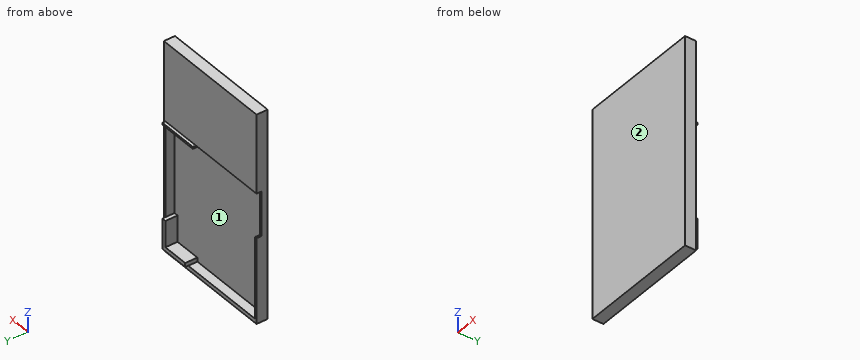
Autodesk Inventor part; units mm, degrees
ref_plane "YZ Plane" through (0, 0, 0) normal (1, 0, 0) x (0, 1, 0)
ref_plane "XZ Plane" through (0, 0, 0) normal (0, 1, 0) x (-1, 0, 0)
ref_plane "XY Plane" through (0, 0, 0) normal (0, 0, 1) x (1, 0, 0)
sketch "Sketch1" plane through (0, 0, 0) normal (0, 1, 0) x (-1, 0, 0)
  line L0 (32.9806, 40.5565) -> (-27.7594, 40.5565)
  line L1 (-27.7594, 40.5565) -> (-27.7594, -62.7415)
  line L2 (-27.7594, -62.7415) -> (32.9806, -62.7415)
  line L3 (32.9806, -62.7415) -> (32.9806, 40.5565)
  point P0 (0, 0)
  dimension "d0" = 60.74
  dimension "d1" = 103.298
extrude "Extrusion1" add sketch "Sketch1" along normal blind 1
sketch "Sketch2" plane through (0, 1, 0) normal (0, 1, 0) x (1, 0, 0)
  line L0 (-32.9806, 62.7415) -> (-32.9806, -40.5565)
  line L1 (27.7594, -40.5565) -> (27.7594, 62.7415)
  line L2 (-32.9806, -40.5565) -> (27.7594, -40.5565)
  line L3 (27.7594, -40.5565) -> (27.7594, -1.5565)
  line L4 (27.7594, -1.5565) -> (-32.9806, -1.5565)
  line L5 (-32.9806, -1.5565) -> (-32.9806, -40.5565)
  point P0 (0, 0)
  point P1 (-32.9806, -1.5565)
  dimension "d4" = 39
extrude "Extrusion2" add sketch "Sketch2" along normal blind 4.5
sketch "Sketch3" plane through (0, 1, 0) normal (0, 1, 0) x (1, 0, 0)
  line L0 (27.7594, -1.5565) -> (-32.9806, -1.5565)
  line L1 (27.7594, 62.7415) -> (-32.9806, 62.7415)
  line L2 (-32.9806, -1.5565) -> (-31.9806, -1.5565)
  line L3 (-31.9806, -1.5565) -> (-31.9806, 62.7415)
  line L4 (-31.9806, 62.7415) -> (-32.9806, 62.7415)
  line L5 (-32.9806, 62.7415) -> (-32.9806, -1.5565)
  line L6 (-31.9806, 62.7415) -> (27.7594, 62.7415)
  line L7 (27.7594, 62.7415) -> (27.7594, 60.7415)
  line L8 (27.7594, 60.7415) -> (-31.9806, 60.7415)
  line L9 (-31.9806, 60.7415) -> (-31.9806, 62.7415)
  line L10 (27.7594, -40.5565) -> (27.7594, 62.7415)
  line L11 (27.7594, -1.5565) -> (26.7594, -1.5565)
  line L12 (26.7594, -1.5565) -> (26.7594, 60.7415)
  line L13 (26.7594, 60.7415) -> (27.7594, 60.7415)
  line L14 (27.7594, 60.7415) -> (27.7594, -1.5565)
  line L15 (-32.9806, -1.5565) -> (-31.9806, -1.5565)
  line L16 (-31.9806, -1.5565) -> (-31.9806, 20.4435)
  line L17 (-31.9806, 20.4435) -> (-32.9806, 20.4435)
  line L18 (-32.9806, 20.4435) -> (-32.9806, -1.5565)
  point P0 (0, 0)
  point P1 (27.2594, -1.5565)
  point P2 (-31.9806, 60.7415)
  point P3 (-32.4806, -1.5565)
  point P4 (-32.4806, 20.4435)
  dimension "d7" = 1
  dimension "d8" = 2
  dimension "d9" = 1
  dimension "d10" = 0
  dimension "d13" = 22
extrude "Extrusion3" add sketch "Sketch3" along normal blind 4.5 contours L0 L12 L8 L10 | L8 L3 L1 L7 | L17 L5 L1 L3
sketch "Sketch4" plane through (0, 1, 0) normal (0, 1, 0) x (1, 0, 0)
  line L0 (-32.9806, 62.7415) -> (-32.9806, -40.5565)
  line L1 (-31.9806, 20.4435) -> (-32.9806, 20.4435)
  line L2 (-32.9806, 20.4435) -> (-32.9806, -2.617)
  line L3 (-32.9806, -2.617) -> (-31.9806, -2.617)
  line L4 (-31.9806, -2.617) -> (-31.9806, 20.4435)
  point P0 (0, 0)
extrude "Extrusion4" add sketch "Sketch4" along normal blind 2
sketch "Sketch5" plane through (0, 1, 0) normal (0, 1, 0) x (1, 0, 0)
  line L0 (26.7594, 60.7415) -> (26.7594, -1.5565)
  line L1 (26.7594, 60.7415) -> (11.7594, 60.7415)
  line L2 (11.7594, 60.7415) -> (11.7594, 58.7415)
  line L3 (11.7594, 58.7415) -> (26.7594, 58.7415)
  line L4 (26.7594, 58.7415) -> (26.7594, 60.7415)
  line L5 (26.7594, 60.7415) -> (24.7594, 60.7415)
  line L6 (24.7594, 60.7415) -> (24.7594, 45.7415)
  line L7 (24.7594, 45.7415) -> (26.7594, 45.7415)
  line L8 (26.7594, 45.7415) -> (26.7594, 60.7415)
  line L9 (26.7594, -1.5565) -> (6.7594, -1.5565)
  line L10 (6.7594, -1.5565) -> (6.7594, -0.5565)
  line L11 (6.7594, -0.5565) -> (26.7594, -0.5565)
  line L12 (26.7594, -0.5565) -> (26.7594, -1.5565)
  point P0 (0, 0)
  point P1 (26.7594, 59.7415)
  point P2 (11.7594, 59.7415)
  point P3 (25.7594, 45.7415)
  point P4 (25.7594, 60.7415)
  point P5 (26.7594, -1.0565)
  point P6 (6.7594, -1.0565)
  point P7 (24.7594, 58.7415)
  dimension "d16" = 2
  dimension "d17" = 15
  dimension "d18" = 2
  dimension "d19" = 15
  dimension "d20" = 1
  dimension "d21" = 20
extrude "Extrusion5" add sketch "Sketch5" along normal blind 6
properties part number "Lid bottom"
For this review, take the finished solid that the model builds, in its own axes (mm). Face numbers are marked on the shaded views. Give positions to 0.01 mm unless a question says otherwise; leave off trailing zeros. Order: outer loops, then holes, each group sorted by start corner. A loop starts at its lowest first (then second) coordinate and runs counter-clockwise, first axis right, second up. Notation, with made-up numbers: (60, 64.25) - (100, 64.25) arc R23 ccw to (100, 83.25) - close; hole circle Ø2 at (1.25, 30.5). An arc over 180 degrees is marked (long way). Answer as a JSON object with one key per item and string values. Group by question number.
Item 1: Take a section at C-C on z = -32.5. Give the boundary of the cut face in (x, y), and give its area (3 significant figures).
Item 2: Clearance check with a flat-ended pin moving along its axis: pin 1 Ø0.5 at (x, z) = (-32.5, -9) entering from +Y. State where the tip first meets the part, or that it passes through.
Item 3: Take a section at B-B on y = 4.25. Give the boundary of the cut face in (x, z).
Item 4: Wall thickness on line 1 along Z through (x, y) = (-25, 1.5); line 2 along X through (y, z) = (2.25, -1.5); line 3 along Z through (x, y) = (20, 6): over which ranges is each line inside the solid? List them lowest first.
Item 5: Take a section at D-D on x = 23. Give the boundary of the cut face in (y, z).
Item 6: Take a section at A-A on x = -26. Give the boundary of the cut face in (y, z), and give its area (3 significant figures).
Item 7: Draft analysis for pull direction Z (two halves, no side actions). For the marked faces 1 and 2, state which applies: pulls with the +Z half, pulls with the -Z half, needs draft (parallel to the pull), parting line crosses it, or undercut.
Reported:
{
 "1": {"outline": "(-32.98, 0) - (27.76, 0) - (27.76, 5.5) - (26.76, 5.5) - (26.76, 1) - (-31.98, 1) - (-31.98, 5.5) - (-32.98, 5.5) - close", "area": "69.7 mm^2"},
 "2": {"pin 1": "y = 3"},
 "3": {"outline": "(-32.98, -62.74) - (27.76, -62.74) - (27.76, 40.56) - (-32.98, 40.56) - (-32.98, 1.56) - (6.76, 1.56) - (6.76, 0.56) - (26.76, 0.56) - (26.76, -45.74) - (24.76, -45.74) - (24.76, -58.74) - (11.76, -58.74) - (11.76, -60.74) - (-31.98, -60.74) - (-31.98, -20.44) - (-32.98, -20.44) - close"},
 "4": {"line 1": "-62.74 to -60.74, 1.56 to 40.56", "line 2": "-32.98 to -31.98, 26.76 to 27.76", "line 3": "-60.74 to -58.74, 0.56 to 1.56"},
 "5": {"outline": "(0, -62.74) - (5.5, -62.74) - (5.5, -60.74) - (7, -60.74) - (7, -58.74) - (1, -58.74) - (1, 0.56) - (7, 0.56) - (7, 1.56) - (5.5, 1.56) - (5.5, 40.56) - (0, 40.56) - close"},
 "6": {"outline": "(0, -62.74) - (5.5, -62.74) - (5.5, -60.74) - (1, -60.74) - (1, 1.56) - (5.5, 1.56) - (5.5, 40.56) - (0, 40.56) - close", "area": "288 mm^2"},
 "7": {"face 1": "undercut", "face 2": "needs draft"}
}
